Verification items for the finished model (mm, model axes). Give positions to 0.01 mm unless a question says otherwise; leave off trailing zeros. Write each loop counter-clockwise with the first axis right and the second up, starting at its lowest first coordinate (ties: lowest second). Pieces come first, ordered by that corner, then holes. Notation, with made-up numbers: M 24.5,-40 L 60.5,-40 A31 ccw 60.5,-12 Z; hole C 63.5,35.5 d9. An arc over 180 degrees is marked long. Answer as a JSON object with one key per item and string values.
```python
from build123d import *

# Parameters (mm, degrees)
F0_W     = 20
F0_H     = 50
F1_DEPTH = 6
F3_D     = 2.5
F5_D     = 2.5


with BuildPart() as f1:
    # F0 (on Front) → F1 (new body)
    with BuildSketch(Plane.XZ):
        with Locations((-10, 25)):
            Rectangle(F0_W, F0_H)
    extrude(amount=F1_DEPTH)

    # F3 (through all)
    with Locations(Plane.XZ.offset(6)):
        with Locations((-5, 45.5), (-5, 4.5), (-15, 14.5), (-15, 35.5)):
            Hole(F3_D / 2)

    # F5 (through all)
    with Locations(Plane(origin=(0, 0, 0), x_dir=(1, 0, 0), z_dir=(0, 1, 0))):
        with Locations((-14, -45.5), (-14, -4.5)):
            Hole(F5_D / 2)


solid = f1.part
```
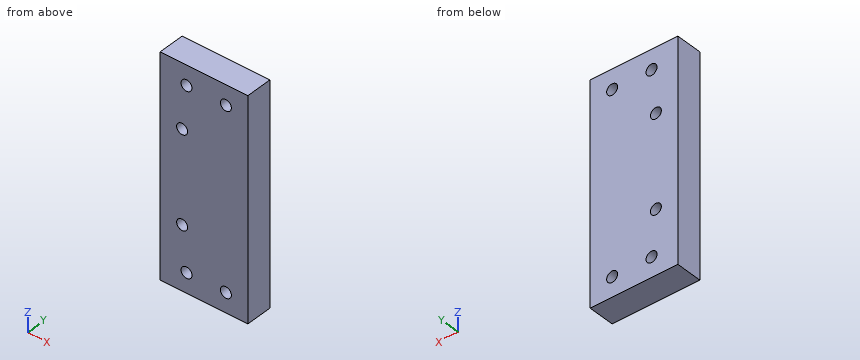
1) Thickness scan on L1, parallel to Z at x = -5, y = -4.25; L2, parallel to Z at x = -14, y = -1.5; L3, parallel to Z at x = -15, y = -2.25. Record the ranges inside material, lowest first.
Completed:
{"L1": "z = 0 to 3.25, 5.75 to 44.25, 46.75 to 50", "L2": "z = 0 to 3.25, 5.75 to 13.75, 15.25 to 34.75, 36.25 to 44.25, 46.75 to 50", "L3": "z = 0 to 3.75, 5.25 to 13.25, 15.75 to 34.25, 36.75 to 44.75, 46.25 to 50"}
2) Section check B-B on y = -4. Record the boundary of the cut face in (x, z), and give its area (3 significant figures).
Completed:
{"outline": "M -20,0 L 0,0 L 0,50 L -20,50 Z; hole C -15,14.5 d2.5; hole C -15,35.5 d2.5; hole C -14,4.5 d2.5; hole C -14,45.5 d2.5; hole C -5,4.5 d2.5; hole C -5,45.5 d2.5", "area": "971 mm2"}
3) Section check A-A on z = 4.5. Record the boundary of the cut face in (x, y), and give its area (3 significant figures).
Completed:
{"outline": "M -20,-6 L -15.25,-6 L -15.25,0 L -20,0 Z; M -12.75,-6 L -6.25,-6 L -6.25,0 L -12.75,0 Z; M -3.75,-6 L 0,-6 L 0,0 L -3.75,0 Z", "area": "90.0 mm2"}
4) Section check D-D on x = -14.75. Record the boundary of the cut face in (y, z), and give its area (3 significant figures).
Completed:
{"outline": "M -6,0 L 0,0 L 0,3.5 L -6,3.5 Z; M -6,5.5 L 0,5.5 L 0,13.28 L -6,13.28 Z; M -6,15.72 L 0,15.72 L 0,34.28 L -6,34.28 Z; M -6,36.72 L 0,36.72 L 0,44.5 L -6,44.5 Z; M -6,46.5 L 0,46.5 L 0,50 L -6,50 Z", "area": "247 mm2"}
5) Go/stop test with a flat-tipped pin: pin 1 (2 mm diameter, centred on x = -5, z = 45.5, fed in from -Y). Record where the tip stops, or that it passes through.
Completed:
{"pin 1": "passes through"}
6) Section check C-C on z = 35.5. Record the boundary of the cut face in (x, y), and give its area (3 significant figures).
Completed:
{"outline": "M -20,-6 L -16.25,-6 L -16.25,0 L -20,0 Z; M -13.75,-6 L 0,-6 L 0,0 L -13.75,0 Z", "area": "105 mm2"}
